Source: three-view drawing plus pictorial views. Frame: mm from the lowest corner of the part. A direction names the side the tool comes from. Coordinates: 2 decimals unless noted, no trailing zeros. Write each loop counter-clockwise with the first axis right and the second up, starting at its lowest first coordinate (ties: lowest second). Pieces come first, ordered by that corner, then holes. Notation, with made-up numbers: (84.25, 13.25) - (128.25, 13.25) arc R33 ccw to (128.25, 44.25) - close; hole circle Ø10 at (-30.5, -8.5). An arc over 180 degrees is marked (long way). One line per item, written item: value.
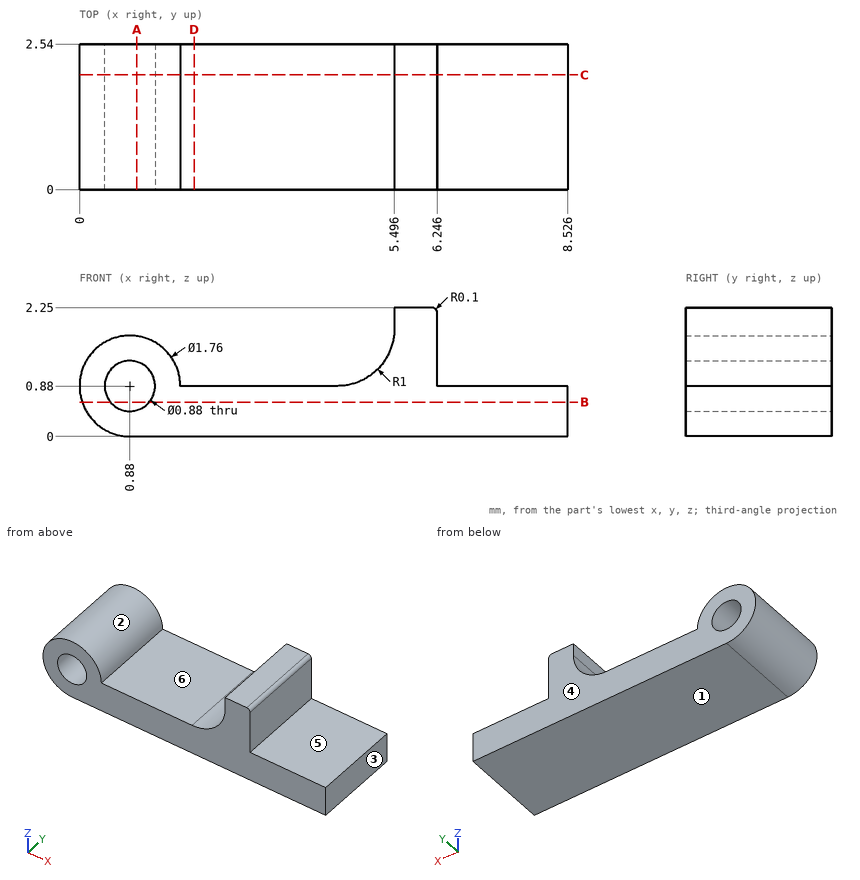
1) Section query D-D on x = 2. Output: boundary loops of the cut face in (y, z).
Values found:
outline: (0, 0) - (2.54, 0) - (2.54, 0.88) - (0, 0.88) - close
2) Reachability of the marked faces 4, 5 and 6 from +Z, -Z, +X, -X, +Y, -Y: full face, straight path, thin tool, end or side. Return the list, or none.
Values found:
face 4: +Z, -Z, +X, -X, +Y
face 5: +Z, +X, +Y, -Y
face 6: +Z, +Y, -Y
3) Material intervals for line 1 (Z direction, x = 8, y = 1.7); line 2 (X direction, y = 0.9, z = 2.1); line 3 (X direction, y = 0.15, z = 0.8), sorted ascending.
Values found:
line 1: 0 to 0.88
line 2: 5.5 to 6.25
line 3: 0 to 0.45, 1.31 to 8.53
4) Section query C-C on y = 2. Output: boundary loops of the cut face in (x, z).
Values found:
outline: (0.88, 0) - (8.53, 0) - (8.53, 0.88) - (6.25, 0.88) - (6.25, 2.15) arc R0.1 ccw to (6.15, 2.25) - (5.5, 2.25) - (5.5, 1.88) arc R1 cw to (4.5, 0.88) - (1.76, 0.88) arc R0.88 ccw (long way) to start; hole circle Ø0.88 at (0.88, 0.88)
5) Section query B-B on z = 0.6. Output: boundary loops of the cut face in (x, y).
Values found:
outline: (0.05, 0) - (0.54, 0) - (0.54, 2.54) - (0.05, 2.54) - close; (1.22, 0) - (8.53, 0) - (8.53, 2.54) - (1.22, 2.54) - close
6) Draft query along X for the marked faces 1, 2 and 3. Return one class per face: released by +X, released by -X, zero draft, split by the parting line, or undercut.
Values found:
face 1: zero draft
face 2: undercut
face 3: released by +X
7) Section query A-A on x = 1. Output: boundary loops of the cut face in (y, z).
Values found:
outline: (0, 0) - (2.54, 0) - (2.54, 0.46) - (0, 0.46) - close; (0, 1.3) - (2.54, 1.3) - (2.54, 1.75) - (0, 1.75) - close
8) Contact query for flat-ended pins moving along their axis: P1, Ø1.1, axis at x = 7, y = 1, coming from the +Z side; P2, Ø1, axis at y = 1, z = 2, coming from the +X side. Output: stop coordinate, or through.
Values found:
P1: z = 0.88
P2: x = 6.25
